Autodesk Inventor part; units mm, degrees
ref_plane "YZ Plane" through (0, 0, 0) normal (1, 0, 0) x (0, 1, 0)
ref_plane "XZ Plane" through (0, 0, 0) normal (0, 1, 0) x (-1, 0, 0)
ref_plane "XY Plane" through (0, 0, 0) normal (0, 0, 1) x (1, 0, 0)
sketch "Skizze1" plane through (0, 0, 0) normal (0, 0, 1) x (1, 0, 0)
  circle A0 centre (0, 0) radius 4
  dimension "d0" = 8
extrude "Extrusion1" add sketch "Skizze1" along normal blind 10
sketch "Skizze2" plane through (0, 0, 10) normal (0, 0, 1) x (1, 0, 0)
  circle A0 centre (0, 0) radius 4
  line L0 (-75, 10) -> (-15, 10)
  arc A1 (-15, 10) -> (-10, 15) centre (-15, 15) ccw
  arc A2 (10, 75) -> (-10, 75) centre (0, 75) ccw
  line L1 (0, -121.8995) -> (0, 121.8995)
  line L2 (-10, 75) -> (-10, 15)
  line L3 (-121.8995, 0) -> (121.8995, 0)
  arc A3 (-75, 10) -> (-85, 0) centre (-75, 0) ccw
  circle A4 centre (0, 75) radius 3.05
  arc A5 (-10, -75) -> (0, -85) centre (0, -75) ccw
  line L4 (-10, -75) -> (-10, -15)
  arc A6 (-10, -15) -> (-15, -10) centre (-15, -15) ccw
  line L5 (-75, -10) -> (-15, -10)
  arc A7 (-75, 10) -> (-75, -10) centre (-75, 0) ccw
  circle A8 centre (-75, 0) radius 3.05
  arc A9 (75, -10) -> (85, 0) centre (75, 0) ccw
  line L6 (75, -10) -> (15, -10)
  arc A10 (15, -10) -> (10, -15) centre (15, -15) ccw
  line L7 (10, -75) -> (10, -15)
  arc A11 (-10, -75) -> (10, -75) centre (0, -75) ccw
  circle A12 centre (0, -75) radius 3.05
  arc A13 (10, 75) -> (0, 85) centre (0, 75) ccw
  line L8 (10, 75) -> (10, 15)
  arc A14 (10, 15) -> (15, 10) centre (15, 15) ccw
  line L9 (75, 10) -> (15, 10)
  arc A15 (75, -10) -> (75, 10) centre (75, 0) ccw
  circle A16 centre (75, 0) radius 3.05
  point P0 (-85, 0)
  point P1 (0, -85)
  point P2 (85, 0)
  point P3 (10, 75)
  dimension "d3" = 10
  dimension "d4" = 5
  dimension "d5" = 10
  dimension "d6" = 75
  dimension "d7" = 75
  dimension "d8" = 6.1
  dimension "d11" = 360
extrude "Extrusion2" add sketch "Skizze2" along normal blind 5 contours L3 L1 A0 | L3 A16 A9 L6 A10 L7 A11 L1 A12 A0 | A0 L1 L3 | A0 L1 A4 A2 L8 A14 L9 A15 L3 A16 | L1 L3 A0 | A0 L3 A8 A3 L0 A1 L2 A2 L1 A4 | L1 A12 A5 L4 A6 L5 A7 L3 A8 A0 | A0 L3 L1
sketch "Skizze3" plane through (0, 0, 15) normal (0, 0, 1) x (1, 0, 0)
  circle A0 centre (0, -75) radius 3.05
  circle A1 centre (75, 0) radius 3.05
  circle A2 centre (0, 75) radius 3.05
  circle A3 centre (-75, 0) radius 3.05
  point P0 (0, 0)
extrude "Extrusion3" add sketch "Skizze3" against normal up to surface (5 mm away)
properties part number "Adapter_Drehteller"
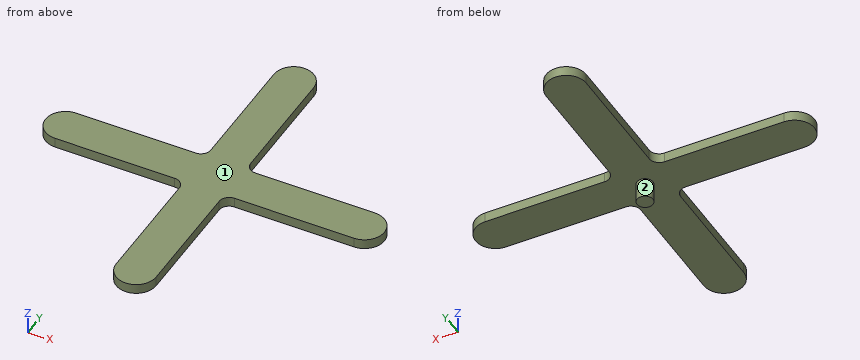
Input: part model. Units: mm. Frame: model coordinates. Face numbers are marked on the shaded views. A direction names the side the tool comes from. Coordinates: 2 decimals unless noted, no trailing zeros. Loops run counter-clockwise (first coordinate to the right, second up) from the corner with the lowest first, then second, coordinate; pieces in that order, holes last. Notation, with made-up numbers: (72, 14.25) -> (130, 14.25) arc R10 ccw to (130, 30.25) -> close; hole circle Ø11 at (-24.5, 80). An arc over 180 degrees is marked (long way). Write each question's results on one line, items separated by ' | '. Start each with the question number.
Q1. Pin query (flat end, axial travel): pin 1 (4 mm diameter, centred on x = -42.5, z = 11.5, fed in from -Y); pin 2 (2.5 mm diameter, centred on y = -40.5, z = 12.5, fed in from +X); pin 3 (5.5 mm diameter, centred on x = -46, z = 13, fed in from +Y). Return the tip coordinate at first contact, or that it passes through.
Q2. Section C-C, the plane y = -45. Return the cut outline in (x, z), plus the area to 3 significant figures.
Q3. Section B-B, the plane x = 0. Return the cut outline in (y, z), plus the area to 3 significant figures.
Q4. Reachability of the marked faces 1 and 2 from +Z, -Z, +X, -X, +Y, -Y: full face, straight path, thin tool, end or side. Return the list, or none.
Q5. Ray query, line 1 (Y direction, x = -32, z = 13.25); line 2 (Z direction, x = 1, y = 19.5). Return the intervals inside material, ascending. Write a range as from..to.
Q6. Section A-A, the plane z = 12. Return the cut outline in (x, y), plus the area to 3 significant figures.
Found:
1) pin 1: y = -10 | pin 2: x = 10 | pin 3: y = 10
2) outline: (-10, 10) -> (10, 10) -> (10, 15) -> (-10, 15) -> close | area: 100 mm2
3) outline: (-85, 10) -> (-4, 10) -> (-4, 0) -> (4, 0) -> (4, 10) -> (85, 10) -> (85, 15) -> (-85, 15) -> close | area: 930 mm2
4) face 1: +Z, +X, -X, +Y, -Y | face 2: -Z
5) line 1: -10..10 | line 2: 10..15
6) outline: (-75, -10) -> (-15, -10) arc R5 cw to (-10, -15) -> (-10, -75) arc R10 ccw to (10, -75) -> (10, -15) arc R5 cw to (15, -10) -> (75, -10) arc R10 ccw to (75, 10) -> (15, 10) arc R5 cw to (10, 15) -> (10, 75) arc R10 ccw to (-10, 75) -> (-10, 15) arc R5 cw to (-15, 10) -> (-75, 10) arc R10 ccw to start | area: 6,250 mm2
